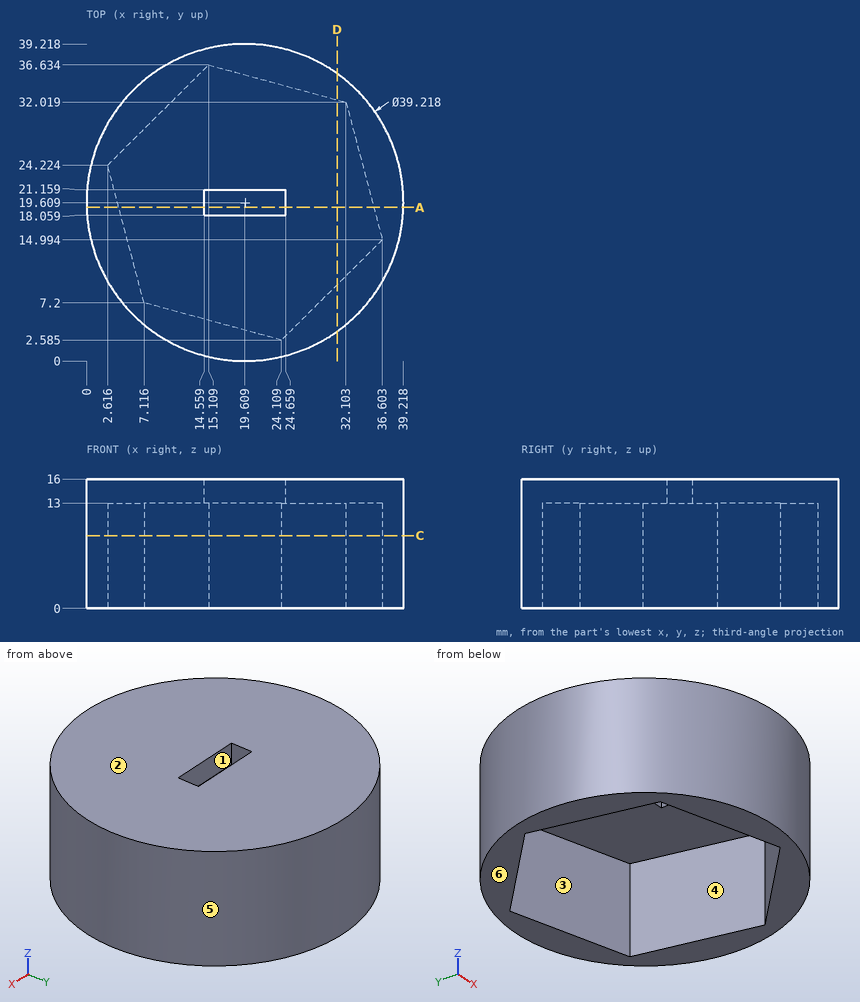
The drawing under review shows one solid part. Ordinate dimensions are in mm from its lowest x, y, z. A direction names the side the tool comes from. Coordinates: 2 decimals unless noted, no trailing zeros. Write each loop counter-clockwise with the first axis right and the second up, starting at its lowest first coordinate (ties: lowest second). Pieces come first, ordered by that corner, then holes. Notation, with made-up numbers: M -30,48.25 L -20,48.25 A24 ccw -20,86.25 Z; hole C 48.5,52 d5. An arc over 180 degrees is marked long. Put each result on its own line as item: value.
1) For the marked faces 1, 2 and 3, list the 3-axis set-ups (+Z, -Z, +X, -X, +Y, -Y) from which the entire face can be reached by the end or side of a thin tool; tool diameter is ignored.
Computed:
face 1: +Z, -Z
face 2: +Z, +X, -X, +Y, -Y
face 3: -Z
2) Draft analysis for pull direction X (two halves, no side actions). For the marked faces 4, 5 and 6, state which applies: released by +X, released by -X, zero draft, split by the parting line, or undercut.
Computed:
face 4: undercut
face 5: split by the parting line
face 6: zero draft
3) Add section D-D on x = 31. Give the boundary of the cut face in (y, z), then the cut area to 3 significant figures.
Computed:
outline: M 3.65,0 L 9.43,0 L 9.43,13 L 32.32,13 L 32.32,0 L 35.57,0 L 35.57,16 L 3.65,16 Z
area: 213 mm2
4) Add section C-C on z = 9. Give the boundary of the cut face in (x, y) (1 decimal).
Computed:
outline: C 19.6,19.6 d39.2; hole M 2.6,24.2 L 7.1,7.2 L 24.1,2.6 L 36.6,15 L 32.1,32 L 15.1,36.6 Z
5) Clearance check with flat-ended pins moving along their axes: pin 1 Ø1 at (x, z) = (6.5, 2) entering from +Y; pin 2 Ø1.5 at (x, z) = (28.5, 14) entering from -Y; pin 3 Ø17 at (x, y) = (12, 21) entering from -Z; pin 4 Ø6 at (x, z) = (21, 8) entering from +Y. State where each tip first meets the part, or that it passes through.
Computed:
pin 1: stops at y = 34.63
pin 2: stops at y = 1.77
pin 3: stops at z = 0
pin 4: stops at y = 39.22
6) Wall thickness on probe 1 along Z at (x, y) = (19, 30); probe 2 along X at (y, z) = (30, 2) (1 decimal); probe 3 along Y at (x, z) = (15.5, 11.5) (1 decimal): over which ranges is each line inside the solid? List them lowest first. Write a range as [from, to].
Computed:
probe 1: z = [13, 16]
probe 2: x = [3, 8.4], [32.6, 36.2]
probe 3: y = [0.4, 4.9], [36.5, 38.8]
7) Add section A-A on y = 19. Give the boundary of the cut face in (x, z).
Computed:
outline: M 0.01,0 L 4,0 L 4,13 L 14.56,13 L 14.56,16 L 0.01,16 Z; M 24.66,13 L 35.54,13 L 35.54,0 L 39.21,0 L 39.21,16 L 24.66,16 Z
